```python
from build123d import *

# Parameters (mm, degrees)
SKIZZE1_R                       = 18.9
SKIZZE1_W                       = 20.3
SKIZZE1_H                       = 20.3
AUFSATZ_LINEAR_AUSTRAGEN1_DEPTH = 21
SKIZZE2_W                       = 20.3
SKIZZE2_H                       = 20.3
AUFSATZ_LINEAR_AUSTRAGEN2_DEPTH = 10
SKIZZE3_R                       = 2.3
SCHNITT_LINEAR_AUSTRAGEN1_DEPTH = 53.412307715
SKETCH1_R                       = 3.75
CUT_EXTRUDE1_DEPTH              = 1.55
CUT_EXTRUDE2_START              = -36.25
SKETCH1_2_R                     = 3.75
CUT_EXTRUDE2_DEPTH              = 1.55
VERRUNDUNG1_R                   = 0.1
VERRUNDUNG2_R                   = 2.5
FASE1_SIZE                      = 0.5
FASE4_SIZE                      = 0.5


with BuildPart() as part:
    # Skizze1 → Aufsatz-Linear austragen1 (new body)
    with BuildSketch(Plane.XY):
        with Locations(Location((0, 0, 0), (0, 0, 180))):
            Circle(SKIZZE1_R)
        Rectangle(SKIZZE1_W, SKIZZE1_H, mode=Mode.SUBTRACT)
    extrude(amount=AUFSATZ_LINEAR_AUSTRAGEN1_DEPTH)

    # Skizze2 → Aufsatz-Linear austragen2 (add)
    with BuildSketch(Plane.XY.offset(21)):
        with BuildLine():
            Line((-14.791551643, 18.9), (14.791551643, 18.9))
            ThreePointArc((14.791551643, 18.9), (16.970562748, 16.970562748), (18.9, 14.791551643))
            Line((18.9, 14.791551643), (18.9, -14.791551643))
            ThreePointArc((18.9, -14.791551643), (16.970562748, -16.970562748), (14.791551643, -18.9))
            Line((14.791551643, -18.9), (-14.791551643, -18.9))
            ThreePointArc((-14.791551643, -18.9), (-16.970562748, -16.970562748), (-18.9, -14.791551643))
            Line((-18.9, -14.791551643), (-18.9, 14.791551643))
            ThreePointArc((-18.9, 14.791551643), (-16.970562748, 16.970562748), (-14.791551643, 18.9))
        make_face()
        Rectangle(SKIZZE2_W, SKIZZE2_H, mode=Mode.SUBTRACT)
    extrude(amount=AUFSATZ_LINEAR_AUSTRAGEN2_DEPTH)

    # Skizze3 → Schnitt-Linear austragen1 (cut, through all)
    with BuildSketch(Plane(origin=(0, 18.9, 0), x_dir=(1, 0, 0), z_dir=(0, 1, 0))):
        with Locations(Location((0, -26, 0), (0, 0, 270))):
            Circle(SKIZZE3_R)
    extrude(amount=-SCHNITT_LINEAR_AUSTRAGEN1_DEPTH, mode=Mode.SUBTRACT)

    # Sketch1 → Cut-Extrude1 (cut)
    with BuildSketch(Plane(origin=(0, 18.9, 0), x_dir=(1, 0, 0), z_dir=(0, 1, 0))):
        with Locations(Location((0, -26, 0), (0, 0, 270))):
            Circle(SKETCH1_R)
    extrude(amount=-CUT_EXTRUDE1_DEPTH, mode=Mode.SUBTRACT)

    # Sketch1<2> → Cut-Extrude2 (cut)
    with BuildSketch(Plane(origin=(0, 18.9, 0), x_dir=(1, 0, 0), z_dir=(0, 1, 0)).offset(CUT_EXTRUDE2_START)):
        with Locations(Location((0, -26, 0), (0, 0, 270))):
            Circle(SKETCH1_2_R)
    extrude(amount=-CUT_EXTRUDE2_DEPTH, mode=Mode.SUBTRACT)

    # Verrundung1
    verrundung1_edges = [part.edges().sort_by_distance(p)[0] for p in [
        (10.15, -10.15, 15.5),
        (10.15, 10.15, 15.5),
        (-10.15, 10.15, 15.5),
        (-10.15, -10.15, 15.5),
    ]]
    fillet(verrundung1_edges, radius=VERRUNDUNG1_R)

    # Verrundung2
    verrundung2_edges = [part.edges().sort_by_distance(p)[0] for p in [
        (-14.791551643, 18.9, 26),
        (-18.9, 14.791551643, 26),
        (-18.9, -14.791551643, 26),
        (-14.791551643, -18.9, 26),
        (14.791551643, -18.9, 26),
        (18.9, -14.791551643, 26),
        (18.9, 14.791551643, 26),
        (14.791551643, 18.9, 26),
    ]]
    fillet(verrundung2_edges, radius=VERRUNDUNG2_R)

    # Fase1
    fase1_edges = [part.edges().sort_by_distance(p)[0] for p in [
        (-16.970562748, -16.970562748, 31),
        (-18.9, 0, 31),
        (-16.970562748, 16.970562748, 31),
        (0, -18.9, 31),
        (16.970562748, -16.970562748, 31),
        (18.9, 0, 31),
        (16.970562748, 16.970562748, 31),
        (0, 18.9, 31),
        (-14.76385305, 18.747066452, 31),
        (-18.747066452, 14.76385305, 31),
        (14.76385305, 18.747066452, 31),
        (18.747066452, 14.76385305, 31),
        (18.747066452, -14.76385305, 31),
        (14.76385305, -18.747066452, 31),
        (-14.76385305, -18.747066452, 31),
        (-18.747066452, -14.76385305, 31),
        (18.9, 0, 0),
        (0, -10.15, 23.7),
        (0, 10.15, 23.7),
        (0, 18.9, 22.25),
        (0, -18.9, 22.25),
        (0, -10.15, 0),
        (0, -10.15, 31),
        (10.15, 0, 0),
        (10.15, 0, 31),
        (-10.15, 0, 0),
        (-10.15, 0, 31),
        (0, 10.15, 0),
        (0, 10.15, 31),
        (10.120710678, -10.120710678, 0),
        (10.120710678, -10.120710678, 31),
        (-10.120710678, -10.120710678, 0),
        (-10.120710678, -10.120710678, 31),
        (-10.120710678, 10.120710678, 0),
        (-10.120710678, 10.120710678, 31),
        (10.120710678, 10.120710678, 0),
        (10.120710678, 10.120710678, 31),
    ]]
    chamfer(fase1_edges, length=FASE1_SIZE)

    # Fase4
    # the kernel refuses this chamfer: 0.5 mm, written as the material it takes off along each edge
    with BuildSketch(Plane(origin=(0, 0, 21), x_dir=(-0.6466454604660656, -0.762790697674421, 0), z_dir=(0.762790697674421, -0.6466454604660656, 0))) as fase4_piece_1:
        Polygon((24, -FASE4_SIZE), (24 - FASE4_SIZE, 0), (24, 0), align=None)
    revolve(axis=Axis((0, 0, 21), (0, 0, -1)), revolution_arc=9.421682318, mode=Mode.SUBTRACT)
    with BuildSketch(Plane(origin=(0, -18.9, 21), x_dir=(0, -0.027495876610589005, 0.9996219169112968), z_dir=(-1, 0, 0))) as fase4_piece_2_section:
        Polygon((FASE4_SIZE * 0.999621916911, FASE4_SIZE * 0.0274958766106), (-FASE4_SIZE * 0.0274958766106, FASE4_SIZE * 0.999621916911), (0, 0), align=None)
    fase4_piece_2 = extrude(amount=13.9028774, mode=Mode.PRIVATE)
    fase4_piece_2 = fase4_piece_2 - Plane(origin=(0, 0, 21.173530337), x_dir=(-1, 0, 0), z_dir=(0, 0, -1)) * Cylinder(18.9, 30, mode=Mode.PRIVATE)
    add(fase4_piece_2, mode=Mode.SUBTRACT)
    with BuildSketch(Plane(origin=(-13.9028774, -16.4, 21), x_dir=(0, -1, 0), z_dir=(1, 0, 0))) as fase4_piece_3:
        Polygon((2.5, -FASE4_SIZE), (2.5 - FASE4_SIZE, 0), (2.5, 0), align=None)
    revolve(axis=Axis((-13.9028774, -16.4, 21), (0, 0, -1)), revolution_arc=40.289158841, mode=Mode.SUBTRACT)
    with BuildSketch(Plane(origin=(-16.4, -13.9028774, 21), x_dir=(-0.7627906976744183, -0.6466454604660687, 0), z_dir=(0.6466454604660687, -0.7627906976744183, 0))) as fase4_piece_4:
        Polygon((2.5, -FASE4_SIZE), (2.5 - FASE4_SIZE, 0), (2.5, 0), align=None)
    revolve(axis=Axis((-16.4, -13.9028774, 21), (0, 0, -1)), revolution_arc=40.289158841, mode=Mode.SUBTRACT)
    with BuildSketch(Plane(origin=(-18.9, 0, 21), x_dir=(-0.027495876610589005, 0, 0.9996219169112968), z_dir=(0, 1, 0))) as fase4_piece_5_section:
        Polygon((FASE4_SIZE * 0.999621916911, FASE4_SIZE * 0.0274958766106), (-FASE4_SIZE * 0.0274958766106, FASE4_SIZE * 0.999621916911), (0, 0), align=None)
    fase4_piece_5 = extrude(amount=13.9028774, mode=Mode.PRIVATE)
    fase4_piece_5 = fase4_piece_5 - Plane(origin=(0, 0, 21.173530342), x_dir=(-1, 0, 0), z_dir=(0, 0, -1)) * Cylinder(18.9, 30, mode=Mode.PRIVATE)
    add(fase4_piece_5, mode=Mode.SUBTRACT)
    with BuildSketch(Plane(origin=(0, 0, 21), x_dir=(0.7627906976744181, -0.646645460466069, 0), z_dir=(0.646645460466069, 0.7627906976744181, 0))) as fase4_piece_6:
        Polygon((24, -FASE4_SIZE), (24 - FASE4_SIZE, 0), (24, 0), align=None)
    revolve(axis=Axis((0, 0, 21), (0, 0, -1)), revolution_arc=9.421682318, mode=Mode.SUBTRACT)
    with BuildSketch(Plane(origin=(18.9, -8.6e-08, 21), x_dir=(0.027495876610589005, 0, 0.9996219169112968), z_dir=(0, -1, 0))) as fase4_piece_7_section:
        Polygon((FASE4_SIZE * 0.999621916911, FASE4_SIZE * 0.0274958766106), (-FASE4_SIZE * 0.0274958766106, FASE4_SIZE * 0.999621916911), (0, 0), align=None)
    fase4_piece_7 = extrude(amount=13.902877314, mode=Mode.PRIVATE)
    fase4_piece_7 = fase4_piece_7 - Plane(origin=(0, 0, 21.173530337), x_dir=(-1, 0, 0), z_dir=(0, 0, -1)) * Cylinder(18.9, 30, mode=Mode.PRIVATE)
    add(fase4_piece_7, mode=Mode.SUBTRACT)
    with BuildSketch(Plane(origin=(16.4, -13.9028774, 21), x_dir=(1, 0, 0), z_dir=(0, 1, 0))) as fase4_piece_8:
        Polygon((2.5, -FASE4_SIZE), (2.5 - FASE4_SIZE, 0), (2.5, 0), align=None)
    revolve(axis=Axis((16.4, -13.9028774, 21), (0, 0, -1)), revolution_arc=40.289158841, mode=Mode.SUBTRACT)
    with BuildSketch(Plane(origin=(13.9028774, -16.4, 21), x_dir=(0.64664546046607, -0.7627906976744174, 0), z_dir=(0.7627906976744174, 0.64664546046607, 0))) as fase4_piece_9:
        Polygon((2.5, -FASE4_SIZE), (2.5 - FASE4_SIZE, 0), (2.5, 0), align=None)
    revolve(axis=Axis((13.9028774, -16.4, 21), (0, 0, -1)), revolution_arc=40.289158841, mode=Mode.SUBTRACT)
    with BuildSketch(Plane(origin=(0, 0, 21), x_dir=(0.6466454604660691, 0.762790697674418, 0), z_dir=(-0.762790697674418, 0.6466454604660691, 0))) as fase4_piece_10:
        Polygon((24, -FASE4_SIZE), (24 - FASE4_SIZE, 0), (24, 0), align=None)
    revolve(axis=Axis((0, 0, 21), (0, 0, -1)), revolution_arc=9.421682318, mode=Mode.SUBTRACT)
    with BuildSketch(Plane(origin=(2.2e-08, 18.9, 21), x_dir=(0, 0.027495876610589005, 0.9996219169112968), z_dir=(1, 0, 0))) as fase4_piece_11_section:
        Polygon((FASE4_SIZE * 0.999621916911, FASE4_SIZE * 0.0274958766106), (-FASE4_SIZE * 0.0274958766106, FASE4_SIZE * 0.999621916911), (0, 0), align=None)
    fase4_piece_11 = extrude(amount=13.902877378, mode=Mode.PRIVATE)
    fase4_piece_11 = fase4_piece_11 - Plane(origin=(0, 0, 21.173530337), x_dir=(-1, 0, 0), z_dir=(0, 0, -1)) * Cylinder(18.9, 30, mode=Mode.PRIVATE)
    add(fase4_piece_11, mode=Mode.SUBTRACT)
    with BuildSketch(Plane(origin=(13.9028774, 16.4, 21), x_dir=(0, 1, 0), z_dir=(-1, 0, 0))) as fase4_piece_12:
        Polygon((2.5, -FASE4_SIZE), (2.5 - FASE4_SIZE, 0), (2.5, 0), align=None)
    revolve(axis=Axis((13.9028774, 16.4, 21), (0, 0, -1)), revolution_arc=40.289158841, mode=Mode.SUBTRACT)
    with BuildSketch(Plane(origin=(16.4, 13.9028774, 21), x_dir=(0.7627906976744174, 0.64664546046607, 0), z_dir=(-0.64664546046607, 0.7627906976744174, 0))) as fase4_piece_13:
        Polygon((2.5, -FASE4_SIZE), (2.5 - FASE4_SIZE, 0), (2.5, 0), align=None)
    revolve(axis=Axis((16.4, 13.9028774, 21), (0, 0, -1)), revolution_arc=40.289158841, mode=Mode.SUBTRACT)
    with BuildSketch(Plane(origin=(0, 0, 21), x_dir=(-0.7627906976744193, 0.6466454604660676, 0), z_dir=(-0.6466454604660676, -0.7627906976744193, 0))) as fase4_piece_14:
        Polygon((24, -FASE4_SIZE), (24 - FASE4_SIZE, 0), (24, 0), align=None)
    revolve(axis=Axis((0, 0, 21), (0, 0, -1)), revolution_arc=9.421682318, mode=Mode.SUBTRACT)
    with BuildSketch(Plane(origin=(-13.9028774, 16.4, 21), x_dir=(0, 1, 0), z_dir=(1, 0, 0))) as fase4_piece_15:
        Polygon((2.5, FASE4_SIZE), (2.5 - FASE4_SIZE, 0), (2.5, 0), align=None)
    revolve(axis=Axis((-13.9028774, 16.4, 21), (0, 0, 1)), revolution_arc=40.289158841, mode=Mode.SUBTRACT)
    with BuildSketch(Plane(origin=(-16.4, 13.9028774, 21), x_dir=(-1, 0, 0), z_dir=(0, -1, 0))) as fase4_piece_16:
        Polygon((2.5, -FASE4_SIZE), (2.5 - FASE4_SIZE, 0), (2.5, 0), align=None)
    revolve(axis=Axis((-16.4, 13.9028774, 21), (0, 0, -1)), revolution_arc=40.289158841, mode=Mode.SUBTRACT)
    with BuildSketch(Plane(origin=(-18.9, -13.9028774, 21), x_dir=(-0.027495876610589005, 0, 0.9996219169112968), z_dir=(0, 1, 0))) as fase4_piece_17_section:
        Polygon((FASE4_SIZE * 0.999621916911, FASE4_SIZE * 0.0274958766106), (-FASE4_SIZE * 0.0274958766106, FASE4_SIZE * 0.999621916911), (0, 0), align=None)
    fase4_piece_17 = extrude(amount=13.9028774, mode=Mode.PRIVATE)
    fase4_piece_17 = fase4_piece_17 - Plane(origin=(0, 0, 21.173530332), x_dir=(-1, 0, 0), z_dir=(0, 0, -1)) * Cylinder(18.9, 30, mode=Mode.PRIVATE)
    add(fase4_piece_17, mode=Mode.SUBTRACT)
    with BuildSketch(Plane(origin=(13.9028774, -18.9, 21), x_dir=(0, -0.027495876610589005, 0.9996219169112968), z_dir=(-1, 0, 0))) as fase4_piece_18_section:
        Polygon((FASE4_SIZE * 0.999621916911, FASE4_SIZE * 0.0274958766106), (-FASE4_SIZE * 0.0274958766106, FASE4_SIZE * 0.999621916911), (0, 0), align=None)
    fase4_piece_18 = extrude(amount=13.9028774, mode=Mode.PRIVATE)
    fase4_piece_18 = fase4_piece_18 - Plane(origin=(0, 0, 21.173530332), x_dir=(-1, 0, 0), z_dir=(0, 0, -1)) * Cylinder(18.9, 30, mode=Mode.PRIVATE)
    add(fase4_piece_18, mode=Mode.SUBTRACT)
    with BuildSketch(Plane(origin=(18.9, 13.9028774, 21), x_dir=(0.027495876610589005, 0, 0.9996219169112968), z_dir=(0, -1, 0))) as fase4_piece_19_section:
        Polygon((FASE4_SIZE * 0.999621916911, FASE4_SIZE * 0.0274958766106), (-FASE4_SIZE * 0.0274958766106, FASE4_SIZE * 0.999621916911), (0, 0), align=None)
    fase4_piece_19 = extrude(amount=13.902877486, mode=Mode.PRIVATE)
    fase4_piece_19 = fase4_piece_19 - Plane(origin=(0, 0, 21.173530332), x_dir=(-1, 0, 0), z_dir=(0, 0, -1)) * Cylinder(18.9, 30, mode=Mode.PRIVATE)
    add(fase4_piece_19, mode=Mode.SUBTRACT)
    with BuildSketch(Plane(origin=(-13.9028774, 18.9, 21), x_dir=(0, 0.027495876610589005, 0.9996219169112968), z_dir=(1, 0, 0))) as fase4_piece_20_section:
        Polygon((FASE4_SIZE * 0.999621916911, FASE4_SIZE * 0.0274958766106), (-FASE4_SIZE * 0.0274958766106, FASE4_SIZE * 0.999621916911), (0, 0), align=None)
    fase4_piece_20 = extrude(amount=13.902877422, mode=Mode.PRIVATE)
    fase4_piece_20 = fase4_piece_20 - Plane(origin=(0, 0, 21.173530342), x_dir=(-1, 0, 0), z_dir=(0, 0, -1)) * Cylinder(18.9, 30, mode=Mode.PRIVATE)
    add(fase4_piece_20, mode=Mode.SUBTRACT)


solid = part.part
```
Source: CAD feature listing. Evaluate the final solid. Frame: model axes, mm. A direction names the side the tool comes from. Coordinates: 2 decimals unless noted, no trailing zeros. Write each loop counter-clockwise with the first axis right and the second up, starting at its lowest first coordinate (ties: lowest second). Pieces come first, ordered by that corner, then holes. Notation, with made-up numbers: (-27, 32.25) -> (-6, 32.25) arc R30 cw to (-6, 64.25) -> close; hole circle Ø4 at (-22.5, 49). An arc over 180 degrees is marked (long way). Return JSON: item names as keys, results as strings. Group by question number.
1) Mould query, pull axis X, two halves, no side actions, for faces 1 (the face through (18.75, -14.75, 26.06)), 2 (the face through (-14, 15, 21)), 3 (the face through (10.15, 0, 15)), 4 (the face through (-2, -17.35, 24)). Classes: +X half, -X half, draft (parallel to the pull), parting line (faces both ways), or undercut.
2) Set-up query: faces 5 (the face through (3.16, 17.88, 28.02)), 6 (the face through (3.16, -17.87, 28.02)), 7 (the face through (13.93, 12.774, 10.853)), 8 (the face through (0, -10.15, 15)). Return all of +Z, -Z, +X, -X, +Y, -Y with unobstructed straight access to the full face (end or side cutting, diameter ignored); none if empty.
3) Section query A-A, the plane z = 11.5. Return loops of the section in (x, y), plus the area to 3 significant figures.
4) Ray query, line 1 along Y through (x, z) = (-7.5, 22.5); line 2 along Y through (x, z) = (-0.5, 23); line 3 along X through (y, z) = (12.5, 26). Return the intervals inside material, ascending.
5) Contact query for flat-ended pins moving along their axis: P1, Ø4, axis at y = -8, z = 5, coming from the -X side; P2, Ø1, axis at x = -11.5, z = 7.5, coming from the +Y side; P3, Ø6, axis at x = 11.5, z = 8, coming from the +Y side. Output: stop coordinate, or through.
From the geometry:
{
 "1": {"face 1": "+X half", "face 2": "draft", "face 3": "undercut", "face 4": "undercut"},
 "2": {"face 5": "+Y", "face 6": "-Y", "face 7": "-Z", "face 8": "+Z, -Z"},
 "3": {"outline": "circle Ø37.8 at (0, 0); hole (-10.15, -10.05) arc R0.1 ccw to (-10.05, -10.15) -> (10.05, -10.15) arc R0.1 ccw to (10.15, -10.05) -> (10.15, 10.05) arc R0.1 ccw to (10.05, 10.15) -> (-10.05, 10.15) arc R0.1 ccw to (-10.15, 10.05) -> close", "area": "710 mm²"},
 "4": {"line 1": "-18.9 to -10.15, 10.15 to 18.9", "line 2": "-17.35 to -10.15, 10.15 to 17.35", "line 3": "-18.9 to -2.3, 2.3 to 18.9"},
 "5": {"P1": "x = -17.92", "P2": "y = 15.37", "P3": "y = 16.88"}
}
